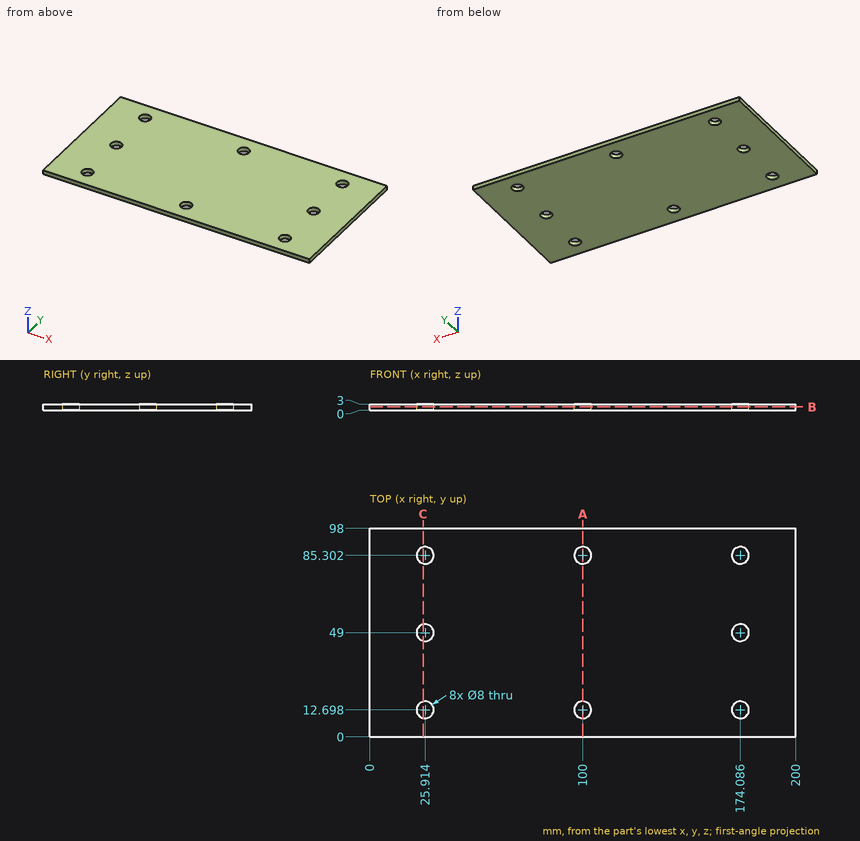
Verification items for this drawing (mm, ordinates from the low corner). Give positions to 0.01 mm unless a question says otherwise; leave off trailing zeros. Loops run counter-clockwise (first coordinate to the right, second up) from the corner with the lowest first, then second, coordinate; pieces in that order, holes last.
1. Material ranges on probe 1 along Y at (x, z) = (100, 1.6); probe 2 along Y at (x, z) = (99, 0.75) (1 decimal); probe 3 along X at (y, z) = (46.5, 0.35), recorded low to high.
Derived:
probe 1: y = 0 to 8.7, 16.7 to 81.3, 89.3 to 98
probe 2: y = 0 to 8.8, 16.6 to 81.4, 89.2 to 98
probe 3: x = 0 to 22.79, 29.04 to 170.96, 177.21 to 200
2. Cross-section at B-B on z = 1.6. Count the separate pieces of the cut face and the enclosed holes in it, and give its area (3 significant figures).
Derived:
separate pieces: 1
enclosed holes: 8
area: 19,200 mm2
3. Cross-section at A-A on x = 100. Record the cut outline in (y, z), and give its area (3 significant figures).
Derived:
outline: (0, 0) - (8.7, 0) - (8.7, 3) - (0, 3) - close; (16.7, 0) - (81.3, 0) - (81.3, 3) - (16.7, 3) - close; (89.3, 0) - (98, 0) - (98, 3) - (89.3, 3) - close
area: 246 mm2
4. Go/stop test with a flat-tipped pin: P1, Ø6.5, axis at x = 25.91, y = 49, coming from the +Z side. Record where the tip stops, or that it passes through.
Derived:
P1: passes through
5. Cross-section at C-C on x = 25. Record the cut outline in (y, z).
Derived:
outline: (0, 0) - (8.8, 0) - (8.8, 3) - (0, 3) - close; (16.59, 0) - (45.11, 0) - (45.11, 3) - (16.59, 3) - close; (52.89, 0) - (81.41, 0) - (81.41, 3) - (52.89, 3) - close; (89.2, 0) - (98, 0) - (98, 3) - (89.2, 3) - close
